```python
from build123d import *

# Parameters (mm, degrees)
SKETCH1_W                                    = 86
SKETCH1_H                                    = 36
BOSS_EXTRUDE1_DEPTH                          = 6.35
CBORE_FOR_M4_HEX_HEAD_CAP_SCREW2_D           = 4.2
CBORE_FOR_M4_HEX_HEAD_CAP_SCREW2_CBORE_D     = 7.6
CBORE_FOR_M4_HEX_HEAD_CAP_SCREW2_CBORE_DEPTH = 4
SKETCH6_R                                    = 1.65
CUT_EXTRUDE1_DEPTH                           = 10


with BuildPart() as part:
    # Sketch1 → Boss-Extrude1 (new, symmetric)
    with BuildSketch(Plane.XY):
        Rectangle(SKETCH1_W, SKETCH1_H)
    extrude(amount=BOSS_EXTRUDE1_DEPTH, both=True)

    # CBORE for M4 Hex Head Cap Screw2 (through all)
    with Locations(Plane(origin=(-8, 8, 6.35), x_dir=(1, 0, 0), z_dir=(0, 0, 1))):
        with Locations((0, 0), (0, -16), (16, -16), (16, 0)):
            CounterBoreHole(CBORE_FOR_M4_HEX_HEAD_CAP_SCREW2_D / 2, CBORE_FOR_M4_HEX_HEAD_CAP_SCREW2_CBORE_D / 2, CBORE_FOR_M4_HEX_HEAD_CAP_SCREW2_CBORE_DEPTH)

    # Sketch6 → Cut-Extrude1 (cut)
    with BuildSketch(Plane.ZY.offset(43)):
        with Locations(Location((0, 14, 0), (0, 0, 270))):
            Circle(SKETCH6_R)
        with Locations(Location((0, -14, 0), (0, 0, 270))):
            Circle(SKETCH6_R)
        with Locations(Location((0, 0, 0), (0, 0, 270))):
            Circle(SKETCH6_R)
    cut_extrude1 = extrude(amount=-CUT_EXTRUDE1_DEPTH, mode=Mode.SUBTRACT)

    # Mirror1: Cut-Extrude1 across plane
    add(cut_extrude1.mirror(Plane(origin=(0, 0, 0), x_dir=(0, 0, 1), z_dir=(1, 0, 0))), mode=Mode.SUBTRACT)


solid = part.part
```
Can you work these out from the model? Positions are in its coordinate system, mm. A direction names the side the tool comes from. Round coordinates to 2 decimals unless told otherwise and drop trailing zeros. Order: outer loops, then holes, each group sorted by start corner. A loop starts at its lowest first (then second) coordinate and runs counter-clockwise, first axis right, second up.
(1) On a 3-axis mill with a long thin cutter (end or side, diameter ignored), from which of +Z, -Z, +X, -X, +Y, -Y can I reach the whole of each face in a straight line? I mean faces 1 (the face through (33, 0, 0)), 2 (the face through (-7.727, 10.082, -2.061)), 3 (the face through (5.2, -5.43, 4.38)), 4 (the face through (-33, 14, 0)). Say none if no direction works.
Results are:
face 1: +X
face 2: +Z, -Z
face 3: +Z
face 4: -X
(2) If we section it at B-B (z = 0): Count the separate pieces of the cut face and the enclosed holes in it, plus the area to 3 significant figures.
Results are:
separate pieces: 1
enclosed holes: 4
area: 2,840 mm2
(3) We'd pull the mould along Y, two halves only. Please class faces 5 (the face through (-1, 18, 0)), 6 (the face through (-7.727, -5.918, -2.061)), 7 (the face through (-43, 0, -3)): +Y half, -Y half, draft (parallel to the pull), parting line (faces both ways), or undercut.
Results are:
face 5: +Y half
face 6: undercut
face 7: draft
(4) If we section it at D-D (x = -37.5): Please give me the cut outline in (y, z), plus the area to 3 significant figures.
Results are:
outline: (-18, -6.35) - (18, -6.35) - (18, 6.35) - (-18, 6.35) - close; hole circle Ø3.3 at (-14, 0); hole circle Ø3.3 at (0, 0); hole circle Ø3.3 at (14, 0)
area: 432 mm2
(5) If we section it at A-A (x = 8): Please give me the cut outline in (y, z), plus the area to 3 significant figures.
Results are:
outline: (-18, -6.35) - (-10.1, -6.35) - (-10.1, 2.35) - (-11.8, 2.35) - (-11.8, 6.35) - (-18, 6.35) - close; (-5.9, -6.35) - (5.9, -6.35) - (5.9, 2.35) - (4.2, 2.35) - (4.2, 6.35) - (-4.2, 6.35) - (-4.2, 2.35) - (-5.9, 2.35) - close; (10.1, -6.35) - (18, -6.35) - (18, 6.35) - (11.8, 6.35) - (11.8, 2.35) - (10.1, 2.35) - close
area: 323 mm2
(6) If we section it at C-C (y = 8): Please give me the cut outline in (x, z).
Results are:
outline: (-43, -6.35) - (-10.1, -6.35) - (-10.1, 2.35) - (-11.8, 2.35) - (-11.8, 6.35) - (-43, 6.35) - close; (-5.9, -6.35) - (5.9, -6.35) - (5.9, 2.35) - (4.2, 2.35) - (4.2, 6.35) - (-4.2, 6.35) - (-4.2, 2.35) - (-5.9, 2.35) - close; (10.1, -6.35) - (43, -6.35) - (43, 6.35) - (11.8, 6.35) - (11.8, 2.35) - (10.1, 2.35) - close
(7) If I drill on L1, parallel to Y at x = -8, z = -1.25; L2, parallel to Y at x = -8, z = 3.95; L3, parallel to Z at x = -38, y = -14, over which ranges is the centre line in solid material (lowest first)?
Results are:
L1: y = -18 to -10.1, -5.9 to 5.9, 10.1 to 18
L2: y = -18 to -11.8, -4.2 to 4.2, 11.8 to 18
L3: z = -6.35 to -1.65, 1.65 to 6.35
(8) I'm going to push a flat-ended pin straight in: pin 1 (2 mm diameter, centred on y = -14, z = 0, fed in from -X). Where does the tip first touch, or does it pass through?
Results are:
pin 1: stops at x = -33
